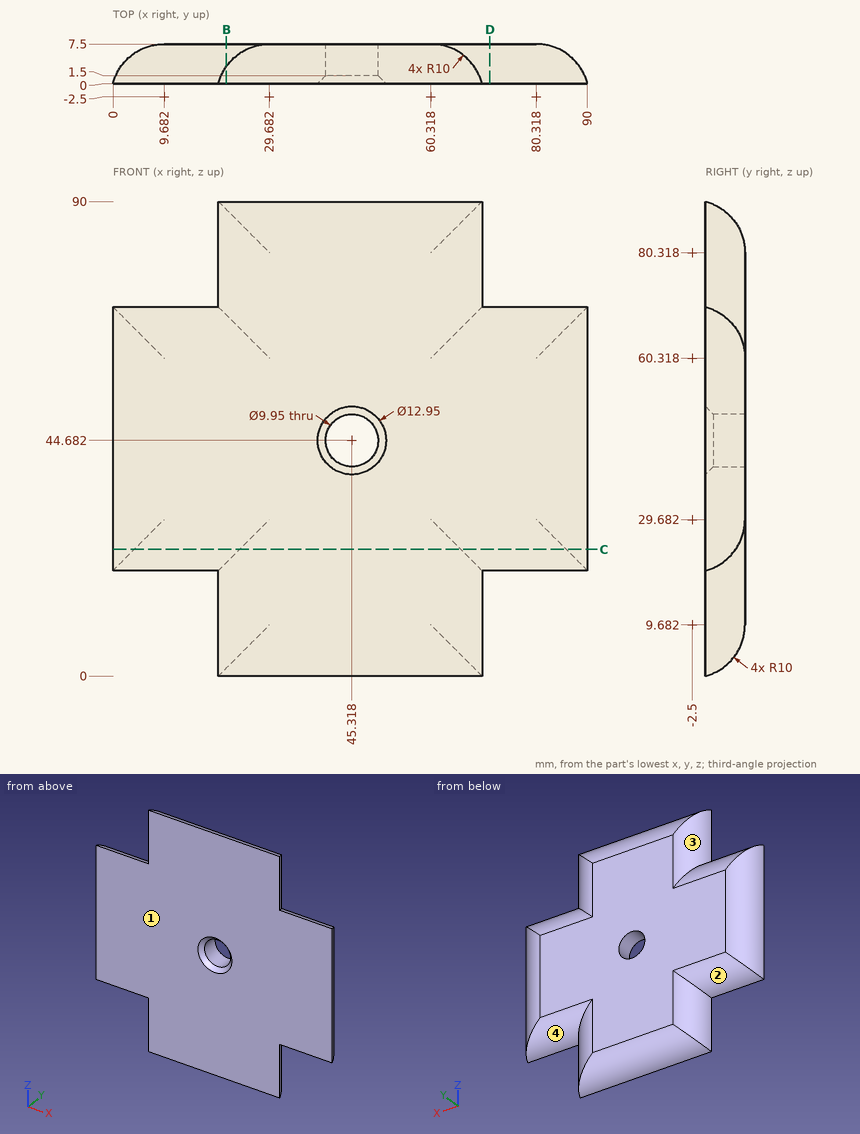
Here's the drawing with two shaded views (mm, measured from the low corner). I have some questions. A direction names the side the tool comes from. Coordinates: 2 decimals unless noted, no trailing zeros. Loops run counter-clockwise (first coordinate to the right, second up) from the corner with the lowest first, then second, coordinate; pieces in that order, holes last. Notation, with made-up numbers: (17.5, 3.25) -> (69.5, 3.25) arc R23 ccw to (69.5, 24.25) -> close; hole circle Ø1 at (-38, 10). An arc over 180 degrees is marked (long way). Answer in a Markdown table with one row per item.
(1) If I drill on probe 1 along Y at (x, z) = (29, 81); probe 2 along Z at (x, y) = (48, 2.75); probe 3 along X at (y, z) = (5, 40.5) (1 decimal), over which ranges is the centre line in solid material (lowest first)?
Results found:
| item | result |
|---|---|
| probe 1 | y = 0 to 7.48 |
| probe 2 | z = 1.17 to 40.49, 48.87 to 88.83 |
| probe 3 | x = 3.1 to 42.6, 48 to 86.9 |
(2) Will these pins go through, and if not, where does the flat tip stop? pin 1 Ø1.5 at (x, y) = (39, 4.5) entering from +Z (1 decimal); pin 2 Ø1.5 at (x, y) = (29.5, 1.5) entering from +Z (1 decimal); pin 3 Ø4 at (y, z) = (6, 44) entering from -X.
Results found:
| item | result |
|---|---|
| pin 1 | stops at z = 88.1 |
| pin 2 | stops at z = 89.8 |
| pin 3 | stops at x = 2.08 |
(3) Imagine slicing it at B-B (x = 21.5). List the corners of the cut face in (y, z) for me, plus the area to 3 significant figures.
Results found:
| item | result |
|---|---|
| outline | (0, 0) arc R10 ccw to (3.25, 1.5) -> (3.25, 21.5) arc R10 ccw to (7.5, 29.68) -> (7.5, 60.32) arc R10 ccw to (3.25, 68.5) -> (3.25, 88.5) arc R10 ccw to (0, 90) -> close |
| area | 467 mm^2 |
(4) Imagine slicing it at C-C (z = 24). List the corners of the cut face in (x, y) for me.
Results found:
| item | result |
|---|---|
| outline | (0, 0) -> (90, 0) arc R10 ccw to (86, 5.73) -> (66, 5.73) arc R10 ccw to (60.32, 7.5) -> (29.68, 7.5) arc R10 ccw to (24, 5.73) -> (4, 5.73) arc R10 ccw to start |
(5) For the marked faces 1, 2, 3 and 4, which set-ups out of +Z, -Z, +X, -X, +Y, -Y let a thin tool reach every point of the face, with its end or its side?
Results found:
| item | result |
|---|---|
| face 1 | +Z, -Z, +X, -X, -Y |
| face 2 | -Z, -X, +Y |
| face 3 | +Z, -X, +Y |
| face 4 | -Z, +X, +Y |
(6) Imagine slicing it at D-D (x = 71.5). List the corners of the cut face in (y, z) for me, plus the area to 3 significant figures.
Results found:
| item | result |
|---|---|
| outline | (0, 20) arc R10 ccw to (7.5, 29.68) -> (7.5, 60.32) arc R10 ccw to (0, 70) -> close |
| area | 337 mm^2 |
